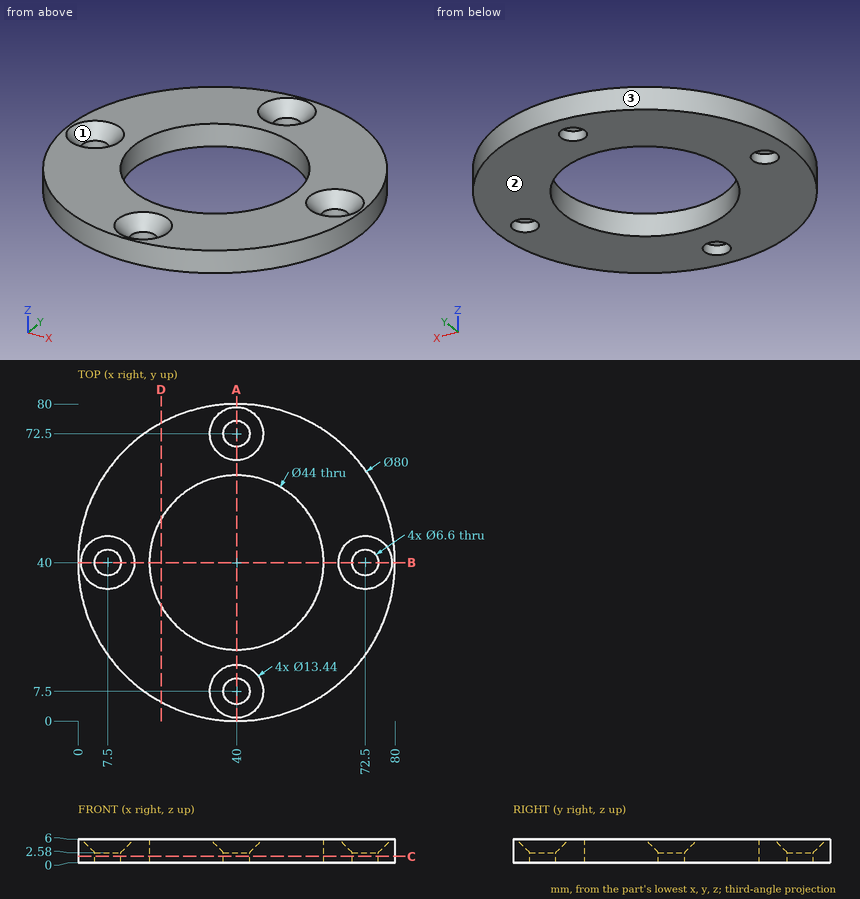
Input: dimensioned drawing with shaded views. Units: mm. Origin: part minimum x, y, z. Give positions to 0.01 mm unless a question says otherwise; leave off trailing zeros. Write each loop counter-clockwise with the first axis right and the second up, starting at its lowest first coordinate (ties: lowest second). Pieces come first, ordered by that corner, then holes.
1. Line query: probe 1 along Y at (x, z) = (40, 1.1); probe 2 along Y at (x, z) = (41, 1.85); probe 3 along X at (y, z) = (72.5, 1.1). Output: solid intervals per line, ascending.
2. Draft query along X for the marked faces 1, 2 and 3. Return one class per face: released by +X, released by -X, zero draft, split by the parting line, or undercut.
3. Pin query (flat end, axial travel): P1, Ø7.5, axis at x = 72.5, y = 40, coming from the +Z side; P2, Ø3, axis at x = 25.5, z = 3.5, coming from the +Y side; P3, Ø1.5, axis at x = 18.5, z = 4.5, coming from the -Y side; P4, Ø5.5, axis at x = 40, y = 7.5, coming from the -Z side. Return the tip coordinate at first contact, or that it passes through.
4. Section query C-C, the plane z = 1.6. Return loops of the section in (x, y).
5. Section query D-D, the plane x = 21. Return loops of the section in (y, z), then the cut area to 3 significant figures.
6. Section query A-A, the plane x = 40. Return loops of the section in (y, z).
Computed:
1. probe 1: y = 0 to 4.2, 10.8 to 18, 62 to 69.2, 75.8 to 80
1. probe 2: y = 0.01 to 4.36, 10.64 to 18.02, 61.98 to 69.36, 75.64 to 79.99
1. probe 3: x = 16.68 to 36.7, 43.3 to 63.32
2. face 1: undercut
2. face 2: zero draft
2. face 3: split by the parting line
3. P1: stops at z = 3.03
3. P2: stops at y = 77.83
3. P3: stops at y = 5.8
3. P4: passes through
4. outline: circle Ø80 at (40, 40); hole circle Ø6.6 at (7.5, 40); hole circle Ø44 at (40, 40); hole circle Ø6.6 at (40, 7.5); hole circle Ø6.6 at (40, 72.5); hole circle Ø6.6 at (72.5, 40)
5. outline: (4.8, 0) - (28.91, 0) - (28.91, 6) - (4.8, 6) - close; (51.09, 0) - (75.2, 0) - (75.2, 6) - (51.09, 6) - close
5. area: 289 mm2
6. outline: (0, 0) - (4.2, 0) - (4.2, 2.58) - (0.78, 6) - (0, 6) - close; (10.8, 0) - (18, 0) - (18, 6) - (14.22, 6) - (10.8, 2.58) - close; (62, 0) - (69.2, 0) - (69.2, 2.58) - (65.78, 6) - (62, 6) - close; (75.8, 0) - (80, 0) - (80, 6) - (79.22, 6) - (75.8, 2.58) - close
